Read the model definition and answer for the solid it produces. Units are mm, in the model's axes. A direction names the side the tool comes from. Give positions to 0.01 mm unless a question says otherwise; leave off trailing zeros. Write each loop counter-clockwise with the first axis right and the second up, starting at its lowest first coordinate (ties: lowest second). Pieces come first, ordered by that corner, then holes.
```python
from build123d import *

# Parameters (mm, degrees)
SKETCH1_W           = 33.3375
SKETCH1_H           = 33.3375
BOSS_EXTRUDE1_DEPTH = 2
SKETCH2_W           = 7.736083449
SKETCH2_H           = 9.461345449
BOSS_EXTRUDE2_DEPTH = 5
SKETCH4_W           = 2.947854253
SKETCH4_H           = 6.435986303
BOSS_EXTRUDE3_DEPTH = 3
SKETCH5_W           = 1.093391386
SKETCH5_H           = 2.729545453
SKETCH5_W_2         = 1.056992946
BOSS_EXTRUDE4_DEPTH = 1
SKETCH6_W           = 7.46808346
SKETCH6_H           = 5.505379369
BOSS_EXTRUDE5_DEPTH = 3


with BuildPart() as part:
    # Sketch1 → Boss-Extrude1 (new body)
    with BuildSketch(Plane(origin=(0, 0, 0), x_dir=(1, 0, 0), z_dir=(0, 1, 0))):
        with Locations((16.66875, 16.66875)):
            Rectangle(SKETCH1_W, SKETCH1_H)
    extrude(amount=BOSS_EXTRUDE1_DEPTH)

    # Sketch2 → Boss-Extrude2 (add)
    with BuildSketch(Plane(origin=(0, 2, 0), x_dir=(1, 0, 0), z_dir=(0, 1, 0))):
        with Locations((6.067363874, 20.718036439)):
            Rectangle(SKETCH2_W, SKETCH2_H)
    extrude(amount=BOSS_EXTRUDE2_DEPTH)

    # Sketch4 → Boss-Extrude3 (add)
    with BuildSketch(Plane(origin=(0, 2, 0), x_dir=(1, 0, 0), z_dir=(0, 1, 0))):
        with Locations((30.638118597, 21.689837472)):
            Rectangle(SKETCH4_W, SKETCH4_H)
    extrude(amount=BOSS_EXTRUDE3_DEPTH)

    # Sketch5 → Boss-Extrude4 (add)
    with BuildSketch(Plane(origin=(0, 2, 0), x_dir=(1, 0, 0), z_dir=(0, 1, 0))):
        with Locations((14.375478356, 30.708236471)):
            Rectangle(SKETCH5_W, SKETCH5_H)
        with Locations((16.871379042, 30.708236471)):
            Rectangle(SKETCH5_W_2, SKETCH5_H)
    extrude(amount=BOSS_EXTRUDE4_DEPTH)

    # Sketch6 → Boss-Extrude5 (add)
    with BuildSketch(Plane(origin=(0, 2, 0), x_dir=(1, 0, 0), z_dir=(0, 1, 0))):
        with Locations((23.229569505, 30.584810316)):
            Rectangle(SKETCH6_W, SKETCH6_H)
    extrude(amount=BOSS_EXTRUDE5_DEPTH)


solid = part.part
```
Item 1: Section C-C (z = -19) is taken. Write down the section's boundary in (x, y).
Result set:
outline: (0, 0) - (33.34, 0) - (33.34, 2) - (32.11, 2) - (32.11, 5) - (29.16, 5) - (29.16, 2) - (9.94, 2) - (9.94, 7) - (2.2, 7) - (2.2, 2) - (0, 2) - close
Item 2: Section D-D (x = 31) is taken. Write down the section's boundary in (y, z).
Result set:
outline: (0, -33.34) - (2, -33.34) - (2, -24.91) - (5, -24.91) - (5, -18.47) - (2, -18.47) - (2, 0) - (0, 0) - close
Item 3: Section A-A (y = 4.25) is taken. Write down the section's boundary in (x, z), and give its area (3 significant figures).
Result set:
outline: (2.2, -25.45) - (9.94, -25.45) - (9.94, -15.99) - (2.2, -15.99) - close; (19.5, -33.34) - (26.96, -33.34) - (26.96, -27.83) - (19.5, -27.83) - close; (29.16, -24.91) - (32.11, -24.91) - (32.11, -18.47) - (29.16, -18.47) - close
area: 133 mm2
Item 4: Section B-B (x = 9) is taken. Write down the section's boundary in (y, z), and give its area (3 significant figures).
Result set:
outline: (0, -33.34) - (2, -33.34) - (2, -25.45) - (7, -25.45) - (7, -15.99) - (2, -15.99) - (2, 0) - (0, 0) - close
area: 114 mm2
Item 5: Which of the six approach directions +Z, -Z, +X, -X, +Y, -Y give full straight-line access (tool end or side, diameter ignored) to faces 1 (the flat face through (14.4, 2.5, -32.073)), 2 (the flat face through (6, 4, -25.449)), 3 (the flat face through (17, 3, -31))?
Result set:
face 1: -Z, -X, +Y
face 2: -Z, +X, -X, +Y
face 3: +Z, -Z, -X, +Y
Item 6: Determine the mould class of faces 4 (the flat face through (6, 7, -21)), 5 (the flat face through (16.343, 2.5, -30.7)), 6 (the flat face through (14.922, 2.5, -30.7)), 7 (the flat face through (2.199, 4, -21)) for opening direction X: pulls with the +X half, pulls with the -X half, needs draft (parallel to the pull), parting line crosses it, or undercut.
Result set:
face 4: needs draft
face 5: undercut
face 6: undercut
face 7: pulls with the -X half
Item 7: Each of these flat-tipped pins is pushed along its axis until it touches: pin 1 Ø0.8 at (y, z) = (2.5, -31.5) entering from +X; pin 2 Ø0.9 at (x, y) = (30.5, 3.5) entering from -Z; pin 3 Ø8 at (x, z) = (9.5, -24) entering from -Y; pin 4 Ø1 at (y, z) = (3, -5) entering from +X. Where does it stop, or does it pass through?
Result set:
pin 1: stops at x = 26.96
pin 2: stops at z = -24.91
pin 3: stops at y = 0
pin 4: passes through
Item 8: Find the intervals of material crossed by line 1 along Y through (x, z) = (29, -17.5); line 2 along Z through (x, y) = (7.5, 5); line 3 along Y through (x, z) = (31, -19), in increasing order.
Result set:
line 1: y = 0 to 2
line 2: z = -25.45 to -15.99
line 3: y = 0 to 5
